Autodesk Inventor part; units mm, degrees
ref_plane "YZ Plane" through (0, 0, 0) normal (1, 0, 0) x (0, 1, 0)
ref_plane "XZ Plane" through (0, 0, 0) normal (0, 1, 0) x (-1, 0, 0)
ref_plane "XY Plane" through (0, 0, 0) normal (0, 0, 1) x (1, 0, 0)
sketch "Sketch1" plane through (0, 0, 0) normal (1, 0, 0) x (0, 1, 0)
  line L0 (0, 0) -> (25, 0)
  line L1 (25, 0) -> (25, -125)
  line L2 (25, -125) -> (0, -125)
  line L3 (0, -125) -> (0, -123)
  line L4 (0, -123) -> (23, -123)
  line L5 (23, -123) -> (23, -2)
  line L6 (23, -2) -> (0, -2)
  line L7 (0, -2) -> (0, 0)
  dimension "d0" = 2
  dimension "d1" = 2
  dimension "d2" = 125
  dimension "d3" = 25
  dimension "d4" = 2
extrude "Extrusion1" add sketch "Sketch1" along normal blind 100
sketch "Sketch2" plane through (0, 0, -123) normal (0, 0, 1) x (1, 0, 0)
  circle A0 centre (80, 11.5) radius 2.75
  line L0 (0, 23) -> (100, 23)
  line L1 (100, 23) -> (100, 0)
  circle A1 centre (20, 11.5) radius 2.75
  line L2 (0, 0) -> (100, 0)
  line L3 (0, 0) -> (0, 23)
  dimension "d7" = 5.5
  dimension "d8" = 11.5
  dimension "d9" = 20
  dimension "d10" = 5.5
  dimension "d11" = 11.5
  dimension "d12" = 20
extrude "Extrusion2" cut sketch "Sketch2" along normal blind 139.25 and the other way blind 73.375 contours A0 | A1
properties part number "Spacer Extrusion" material "Aluminum 6061"
For this review, take the finished solid that the model builds, in its own axes (mm). A direction names the side the tool comes from. Round coordinates to 2 decimals unless told otherwise and drop trailing zeros. Order: outer loops, then holes, each group sorted by start corner. A loop starts at its lowest first (then second) coordinate and runs counter-clockwise, first axis right, second up.
Q1. We need section B-B, the plane x = 20. Give the boundary of the cut face in (y, z).
Findings below:
outline: (0, -125) - (8.75, -125) - (8.75, -123) - (0, -123) - close; (0, -2) - (8.75, -2) - (8.75, 0) - (0, 0) - close; (14.25, -125) - (25, -125) - (25, 0) - (14.25, 0) - (14.25, -2) - (23, -2) - (23, -123) - (14.25, -123) - close
Q2. Mouldability with a two-part tool opening along Z and no side actions: class faces 3 (the flat face through (49, 13, -125)), 4 (the flat face through (49, 23, -63)), 5 (the flat face through (49, 11, -123)), 6 (the cylindrical face through (17.253, 11.621, -123.986)) as pulls with the +Z half, pulls with the -Z half, needs draft (parallel to the pull), parting line crosses it, or undercut.
Findings below:
face 3: pulls with the -Z half
face 4: undercut
face 5: undercut
face 6: needs draft
Q3. Machinability: for faces 1 (the flat face through (49, 12, -2)), 2 (the flat face through (0, 24, -62)), which of the approach directions +Z, -Z, +X, -X, +Y, -Y give a long, thin tool a straight path to every point of the face, cutting with its end or side? Answer none if there is none.
Findings below:
face 1: +X, -X, -Y
face 2: +Z, -Z, -X, +Y, -Y
Q4. Wall thickness on line 1 (X direction, y = 11.5, z = -0.7); line 2 (Z direction, x = 44, y = 7); line 3 (Y direction, x = 20, z = -124.15): over which ranges is each line inside the solid? List them lowest first.
Findings below:
line 1: x = 0 to 17.25, 22.75 to 77.25, 82.75 to 100
line 2: z = -125 to -123, -2 to 0
line 3: y = 0 to 8.75, 14.25 to 25
Q5. We need section D-D, the plane x = 42. Give the boundary of the cut face in (y, z), plus the area to 3 significant figures.
Findings below:
outline: (0, -125) - (25, -125) - (25, 0) - (0, 0) - (0, -2) - (23, -2) - (23, -123) - (0, -123) - close
area: 342 mm2
Q6. Insertion check: P1, Ø10, axis at x = 13, z = -96, coming from the -Y side. The pin has a flat end and moves straight along its axis. Give the tip position at first contact, or say it passes through.
Findings below:
P1: stops at y = 23
Q7. We need section C-C, the plane y = 4.75. Give the boundary of the cut face in (x, z), plus the area to 3 significant figures.
Findings below:
outline: (0, -125) - (100, -125) - (100, -123) - (0, -123) - close; (0, -2) - (100, -2) - (100, 0) - (0, 0) - close
area: 400 mm2
Q8. We need section A-A, the plane y = 11.5. Give the boundary of the cut face in (x, z).
Findings below:
outline: (0, -125) - (17.25, -125) - (17.25, -123) - (0, -123) - close; (0, -2) - (17.25, -2) - (17.25, 0) - (0, 0) - close; (22.75, -125) - (77.25, -125) - (77.25, -123) - (22.75, -123) - close; (22.75, -2) - (77.25, -2) - (77.25, 0) - (22.75, 0) - close; (82.75, -125) - (100, -125) - (100, -123) - (82.75, -123) - close; (82.75, -2) - (100, -2) - (100, 0) - (82.75, 0) - close
